from build123d import *

# Parameters (mm, degrees)
SKETCH1_W           = 3
SKETCH1_H           = 10
SKETCH1_W_2         = 27.5
SKETCH1_H_2         = 3
SKETCH1_W_3         = 8
SKETCH1_W_4         = 3.5
BOSS_EXTRUDE1_DEPTH = 3


with BuildPart() as part:
    # Sketch1 → Boss-Extrude1 (new body)
    with BuildSketch(Plane.XY):
        with Locations((-29, -15)):
            Rectangle(SKETCH1_W, SKETCH1_H)
        with Locations((-29, -35)):
            Rectangle(SKETCH1_W, SKETCH1_H)
        Polygon((-27.5, -60), (-27.5, -57), (-27.5, -50), (-30.5, -50), (-30.5, -60), align=None)
        Polygon((0, -57), (0, -3), (-3.5, -3), (-11.5, -3), (-19.5, -3), (-27.5, -3), (-27.5, -10), (-27.5, -20), (-27.5, -30), (-27.5, -40), (-27.5, -50), (-27.5, -57), align=None)
        Polygon((27.5, -10), (27.5, -3), (19.5, -3), (11.5, -3), (3.5, -3), (0, -3), (0, -57), (27.5, -57), (27.5, -50), (27.5, -40), (27.5, -30), (27.5, -20), align=None)
        with Locations((-13.75, -58.5)):
            Rectangle(SKETCH1_W_2, SKETCH1_H_2)
        with Locations((13.75, -58.5)):
            Rectangle(SKETCH1_W_2, SKETCH1_H_2)
        Polygon((30.5, -50), (27.5, -50), (27.5, -57), (27.5, -60), (30.5, -60), align=None)
        with Locations((29, -35)):
            Rectangle(SKETCH1_W, SKETCH1_H)
        with Locations((29, -15)):
            Rectangle(SKETCH1_W, SKETCH1_H)
        with Locations((15.5, -1.5)):
            Rectangle(SKETCH1_W_3, SKETCH1_H_2)
        with Locations((1.75, -1.5)):
            Rectangle(SKETCH1_W_4, SKETCH1_H_2)
        with Locations((-1.75, -1.5)):
            Rectangle(SKETCH1_W_4, SKETCH1_H_2)
        with Locations((-15.5, -1.5)):
            Rectangle(SKETCH1_W_3, SKETCH1_H_2)
    extrude(amount=BOSS_EXTRUDE1_DEPTH)


solid = part.part
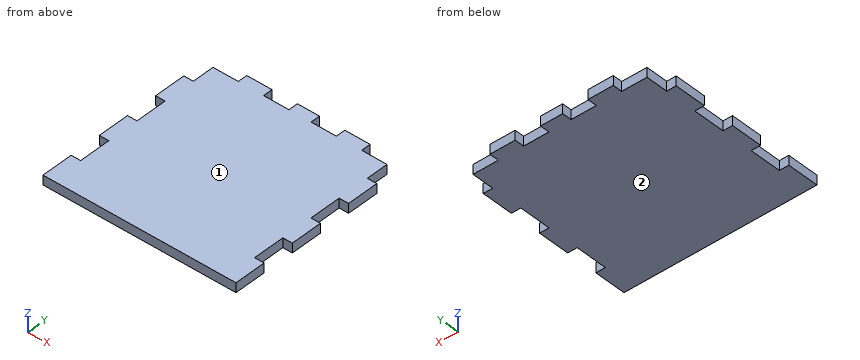
Geometry check sheet. Reference: the model listing, model coordinates, mm. Face numbers are marked on the shaded views. Give positions to 0.01 mm unless a question says otherwise; leave off trailing zeros. Order: outer loops, then holes, each group sorted by start corner. A loop starts at its lowest first (then second) coordinate and runs counter-clockwise, first axis right, second up.
1) Cross-section at B-B (x = 6.5). Record the boundary of the cut face in (y, z).
Results are:
outline: (-60, 0) - (-3, 0) - (-3, 3) - (-60, 3) - close
2) Cross-section at A-A (y = -7.5). Record the boundary of the cut face in (x, z).
Results are:
outline: (-27.5, 0) - (27.5, 0) - (27.5, 3) - (-27.5, 3) - close
3) Material ranges on probe 1 along X at (y, z) = (-41.5, 1.8); probe 2 along Y at (x, z) = (-10, 0.2), recorded low to high.
Results are:
probe 1: x = -27.5 to 27.5
probe 2: y = -60 to -3
4) Gauge pin test, flat ends, axial feed: pin 1 (0.9 mm diameter, centred on x = 23, z = 1, fed in from +Y); pin 2 (0.9 mm diameter, centred on y = -1.5, z = 1.5, fed in from -X); pin 3 (1.5 mm diameter, centred on y = -1, z = 1.5, fed in from +X). Record the tip position at first contact, or that the pin passes through.
Results are:
pin 1: stops at y = -3
pin 2: stops at x = -19.5
pin 3: stops at x = 19.5
5) Draft check along Z on the marked faces 1 and 2. Enter one of: released by +Z, released by -Z, zero draft, split by the parting line, or undercut.
Results are:
face 1: released by +Z
face 2: released by -Z
